Could you check a few things on this drawing? It's one solid part, dimensions in mm from its lowest x, y, z. A direction names the side the tool comes from. Round coordinates to 2 decimals unless told otherwise and drop trailing zeros. Use a Markdown table: item, result. Add a question column.
(1) On a 3-axis mill with a long thin cutter (end or side, diameter ignored), from which of +Z, -Z, +X, -X, +Y, -Y can I reach the whole of each face in a straight line? I mean the marked faces 4, 5 and 6. Say none if no direction works.
(2) If I drill on probe 1 along Y at (x, z) = (31, 7); probe 2 along Z at (x, y) = (31.5, 39.5) (1 decimal); probe 3 along Z at (x, y) = (18, 54.5), over which ranges is the centre line in solid material (lowest first)?
(3) I want a section at A-A, the plane z = 2.5. Give the number of separate pieces and of enclosed holes in the cut face.
(4) I'm going to push flat-ended pins straight in: P1, Ø5, axis at x = 13.5, y = 14, coming from the +Z side; P2, Ø10, axis at x = 31.5, y = 56.5, coming from the +Z side; P3, Ø12, axis at x = 29, y = 55, coming from the -Z side. Where does each tip first touch, or does it pass through?
(5) Thinking about a two-plate mould opening in X: for the marked faces 1, 2 and 3, which applies, pulls with the +X half, pulls with the -X half, needs draft (parallel to the pull), parting line crosses it, or undercut?
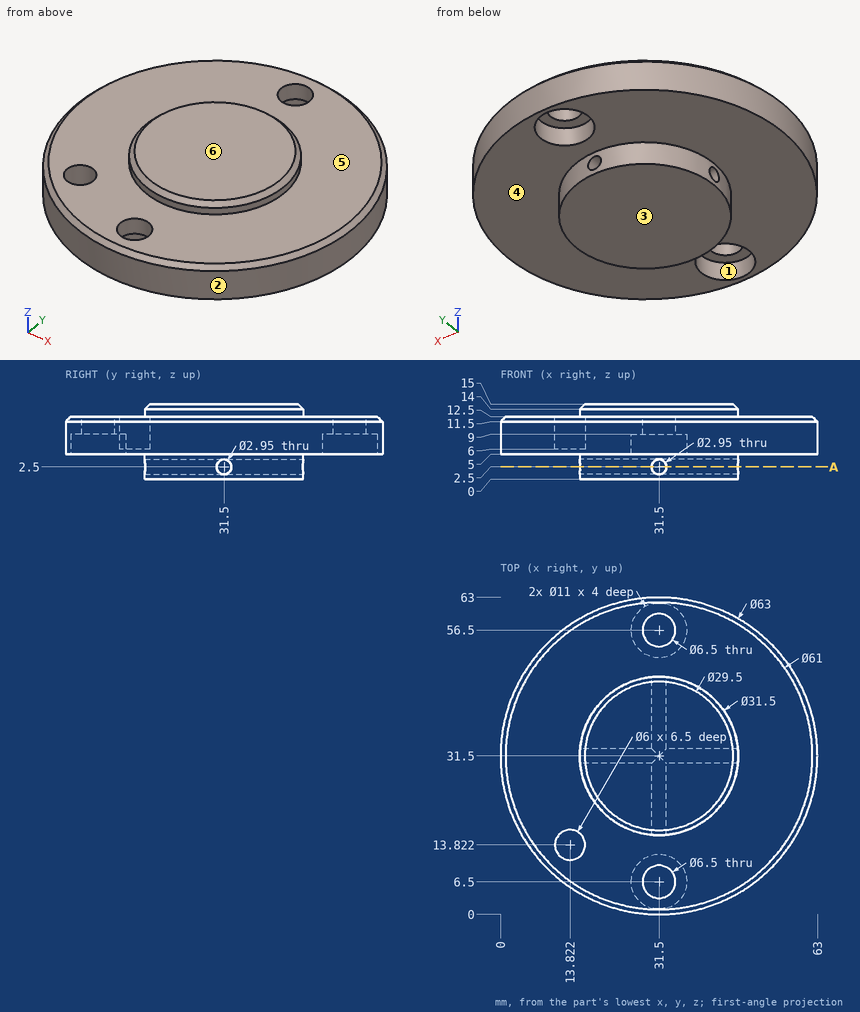
Taken from the geometry:
| question | item | result |
|---|---|---|
| 1 | face 4 | -Z |
| 1 | face 5 | +Z |
| 1 | face 6 | +Z, +X, -X, +Y, -Y |
| 2 | probe 1 | y = 0 to 1.02, 11.98 to 51.02, 61.98 to 63 |
| 2 | probe 2 | z = 0 to 1, 4 to 15 |
| 2 | probe 3 | z = 5 to 12.5 |
| 3 | separate pieces | 4 |
| 3 | enclosed holes | 0 |
| 4 | P1 | stops at z = 6 |
| 4 | P2 | stops at z = 12.5 |
| 4 | P3 | stops at z = 5 |
| 5 | face 1 | undercut |
| 5 | face 2 | parting line crosses it |
| 5 | face 3 | needs draft |
